from build123d import *

# Parameters (mm, degrees)
BOSS_EXTRUDE1_DEPTH = 4.5
SKETCH4_R           = 8.45
BOSS_EXTRUDE2_DEPTH = 18
BOSS_EXTRUDE3_DEPTH = 4.5
SKETCH2_R           = 0.8
CUT_EXTRUDE2_DEPTH  = 6.5
BOSS_EXTRUDE4_DEPTH = 4.5
SKETCH2_2_R         = 0.8
CUT_EXTRUDE4_DEPTH  = 6
CUT_EXTRUDE5_DEPTH  = 16


with BuildPart() as part:
    # Sketch1 → Boss-Extrude1 (new body)
    with BuildSketch(Plane.XY):
        Polygon((5.572251372, 3.818378537), (-0.520687129, 6.734900513), (-6.0929385, 2.916521976), (-5.572251372, -3.818378537), (0.520687129, -6.734900513), (6.0929385, -2.916521976), align=None)
    extrude(amount=BOSS_EXTRUDE1_DEPTH)

    # Sketch4 → Boss-Extrude2 (add)
    with BuildSketch(Plane(origin=(0, 0, 0), x_dir=(-1, 0, 0), z_dir=(0, 0, -1))):
        Circle(SKETCH4_R)
    extrude(amount=BOSS_EXTRUDE2_DEPTH)

    # Sketch1<2> → Boss-Extrude3 (add)
    with BuildSketch(Plane.XY):
        Polygon((5.572251372, 3.818378537), (-0.520687129, 6.734900513), (-6.0929385, 2.916521976), (-5.572251372, -3.818378537), (0.520687129, -6.734900513), (6.0929385, -2.916521976), align=None)
    extrude(amount=BOSS_EXTRUDE3_DEPTH)

    # Sketch2 → Cut-Extrude2 (cut)
    with BuildSketch(Plane.XY.offset(4.5)):
        Circle(SKETCH2_R)
    extrude(amount=-CUT_EXTRUDE2_DEPTH, mode=Mode.SUBTRACT)

    # Sketch1<3> → Boss-Extrude4 (add)
    with BuildSketch(Plane.XY):
        Polygon((5.572251372, 3.818378537), (-0.520687129, 6.734900513), (-6.0929385, 2.916521976), (-5.572251372, -3.818378537), (0.520687129, -6.734900513), (6.0929385, -2.916521976), align=None)
    extrude(amount=BOSS_EXTRUDE4_DEPTH)

    # Sketch2<2> → Cut-Extrude4 (cut)
    with BuildSketch(Plane.XY.offset(4.5)):
        Circle(SKETCH2_2_R)
    extrude(amount=-CUT_EXTRUDE4_DEPTH, mode=Mode.SUBTRACT)

    # Sketch5 → Cut-Extrude5 (cut)
    with BuildSketch(Plane(origin=(0, 0, -18), x_dir=(-1, 0, 0), z_dir=(0, 0, -1))):
        with BuildLine():
            Line((-1.965909199, -1.850729862), (1.965909199, -1.850729862))
            ThreePointArc((1.965909199, -1.850729862), (2.7, 0), (1.965909199, 1.850729862))
            Line((1.965909199, 1.850729862), (-1.965909199, 1.850729862))
            ThreePointArc((-1.965909199, 1.850729862), (-2.7, 0), (-1.965909199, -1.850729862))
        make_face()
    extrude(amount=-CUT_EXTRUDE5_DEPTH, mode=Mode.SUBTRACT)


solid = part.part
Part model, mm, in its own coordinate system. A direction names the side the tool comes from. Give positions to 0.01 mm unless a question says otherwise; leave off trailing zeros. Write each loop counter-clockwise with the first axis right and the second up, starting at its lowest first coordinate (ties: lowest second). Pieces come first, ordered by that corner, then holes.
1) Cut at D-D on y = -4.5. Write the cut outline in (x, z), then the cut area to 3 significant figures.
Resolved:
outline: (-7.15, -18) - (7.15, -18) - (7.15, 0) - (3.78, 0) - (3.78, 4.5) - (-4.15, 4.5) - (-4.15, 0) - (-7.15, 0) - close
area: 293 mm2
2) Cut at C-C on x = 0. Write the cut outline in (y, z), then the cut area to 3 significant figures.
Resolved:
outline: (-8.45, -18) - (-1.85, -18) - (-1.85, -2) - (-0.8, -2) - (-0.8, 4.5) - (-6.49, 4.5) - (-6.49, 0) - (-8.45, 0) - close; (0.8, -2) - (1.85, -2) - (1.85, -18) - (8.45, -18) - (8.45, 0) - (6.49, 0) - (6.49, 4.5) - (0.8, 4.5) - close
area: 293 mm2
3) Two-plate mould, pull along X, no slides. Class faces 4 (the face through (2.7, 0, -10.1)), 5 (the face through (-3.27, 4.85, 2.22)), 6 (the face through (-1, 0, 4.5)): released by +X, released by -X, zero draft, split by the parting line, or undercut.
Resolved:
face 4: undercut
face 5: released by -X
face 6: zero draft
4) Pin check, flat tips, straight feed: pin 1 (4 mm diameter, centred on y = -2.5, z = -9.5, fed in from -X); pin 2 (4 mm diameter, centred on x = 6.5, z = -10.5, fed in from -Y); pin 3 (2 mm diameter, centred on x = 6.5, z = -9, fed in from +Y) (3 decimals). Stop position of each tip, or through.
Resolved:
pin 1: stops at x = -8.44
pin 2: stops at y = -7.15
pin 3: stops at y = 6.415
5) Cut at A-A on y = 0. Write the cut outline in (x, z), then the cut area to 3 significant figures.
Resolved:
outline: (-8.45, -18) - (-2.7, -18) - (-2.7, -2) - (-0.8, -2) - (-0.8, 4.5) - (-5.87, 4.5) - (-5.87, 0) - (-8.45, 0) - close; (0.8, -2) - (2.7, -2) - (2.7, -18) - (8.45, -18) - (8.45, 0) - (5.87, 0) - (5.87, 4.5) - (0.8, 4.5) - close
area: 260 mm2
6) Which spindle directions (+Z, -Z, +X, -X, +Y, -Y) get a long thin tool onto all of the face, cutting with end or side? Do faces 1 (the face through (-5.836, -0.404, 2.218)), 2 (the face through (2.568, 5.256, 2.218)), 3 (the face through (3.27, -4.85, 2.22)). Say none if no direction does.
Resolved:
face 1: +Z, -X, -Y
face 2: +Z, +X, +Y
face 3: +Z, +X, -Y
7) Probe L1, parallel to Y at x = -0.25, z = -4; L2, parallel to Z at x = 5.5, y = 4; L3, parallel to Y at x = 0, z = 1. List the from-to ranges inside material, lowest first.
Resolved:
L1: y = -8.45 to -1.85, 1.85 to 8.45
L2: z = -18 to 0
L3: y = -6.49 to -0.8, 0.8 to 6.49
8) Cut at B-B on z = -6. Write the cut outline in (x, y).
Resolved:
outline: circle Ø16.9 at (0, 0); hole (-1.97, -1.85) - (1.97, -1.85) arc R2.7 ccw to (1.97, 1.85) - (-1.97, 1.85) arc R2.7 ccw to start
